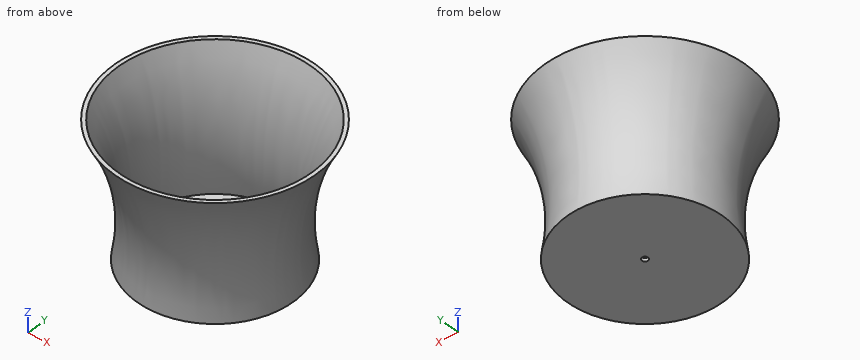
from build123d import *

# Parameters (mm, degrees)
F2_T     = -3
F3_R     = 2.7
F4_DEPTH = 25


with BuildPart() as f1:
    # F0 (on Front) → F1 (revolve)
    with BuildSketch(Plane.XZ):
        with BuildLine():
            Line((-70, 0), (0, 0))
            Line((0, 0), (0, 120))
            Line((0, 120), (-90, 120))
            ThreePointArc((-90, 120), (-69.464997, 61.755834), (-70, 0))
        make_face()
    revolve(axis=Axis((0, 0, 60), (0, 0, 1)))

    # F2
    f2_openings = [f1.faces().sort_by_distance(p)[0] for p in [
        (0, 0, 120),
    ]]
    offset(amount=F2_T, openings=f2_openings)

    # F3 (on face) → F4 (cut)
    with BuildSketch(Plane(origin=(0, 0, 0), x_dir=(1, 0, 0), z_dir=(0, 0, -1))):
        Circle(F3_R)
    extrude(amount=-F4_DEPTH, mode=Mode.SUBTRACT)


solid = f1.part
Geometry check sheet. Reference: the model listing, model coordinates, mm. Round coordinates to 2 decimals unless told otherwise and drop trailing zeros. Order: outer loops, then holes, each group sorted by start corner. A loop starts at its lowest first (then second) coordinate and runs counter-clockwise, first axis right, second up. Notation, with made-up numbers: M 77.5,56 L 107.5,56 A25 cw 107.5,83 Z; hole C -5,29 d10. An arc over 180 degrees is marked long. Answer in a Markdown table with one row per item. Add a question column.
Item 1: Sectioned sample at D-D, the plane z = 91. Enter the section's corners in (x, y).
Item 2: Sectioned sample at C-C, the plane z = 107.5. Enter the section's corners in (x, y).
Item 3: Depth check by flat-ended pin: pin 1 Ø3 at (x, y) = (0, 0) entering from -Z; pin 2 Ø1 at (x, y) = (-58.5, -64) entering from -Z; pin 3 Ø6 at (x, z) = (-42, 64) entering from +Y; pin 4 Ø12 at (y, z) = (5.5, 35.5) entering from +X. Enter the tip coordinate at first touch or a pass-through.
Item 4: Sectioned sample at A-A, the plane x = 0. Enter the section's corners in (y, z).
Item 5: Material ranges on L1, parallel to Z at x = 20, y = -54; L2, parallel to Y at x = 0, z = 1.7; L3, parallel to Y at x = -52.5, z = 91, recorded low to high. Write a range as [from, to].
Filled in:
| question | item | result |
|---|---|---|
| 1 | outline | C 0,0 d153.85; hole C 0,0 d147.5 |
| 2 | outline | C 0,0 d167.19; hole C 0,0 d160.59 |
| 3 | pin 1 | passes through |
| 3 | pin 2 | stops at z = 112.89 |
| 3 | pin 3 | stops at y = 58.06 |
| 3 | pin 4 | stops at x = 67.18 |
| 4 | outline | M -90,120 A178.56 cw -70,0 L -2.7,0 L -2.7,3 L -66.43,3 A181.56 ccw -86.57,120 Z; M 2.7,0 L 70,0 A178.56 cw 90,120 L 86.57,120 A181.56 ccw 66.43,3 L 2.7,3 Z |
| 5 | L1 | z = [0, 3] |
| 5 | L2 | y = [-69.69, -2.7], [2.7, 69.69] |
| 5 | L3 | y = [-56.22, -51.8], [51.8, 56.22] |
